The drawing under review shows one solid part. Ordinate dimensions are in mm from its lowest x, y, z. A direction names the side the tool comes from. Coordinates: 2 decimals unless noted, no trailing zeros. Order: outer loops, then holes, each group sorted by start corner. A loop starts at its lowest first (then second) coordinate and runs counter-clockwise, first axis right, second up.
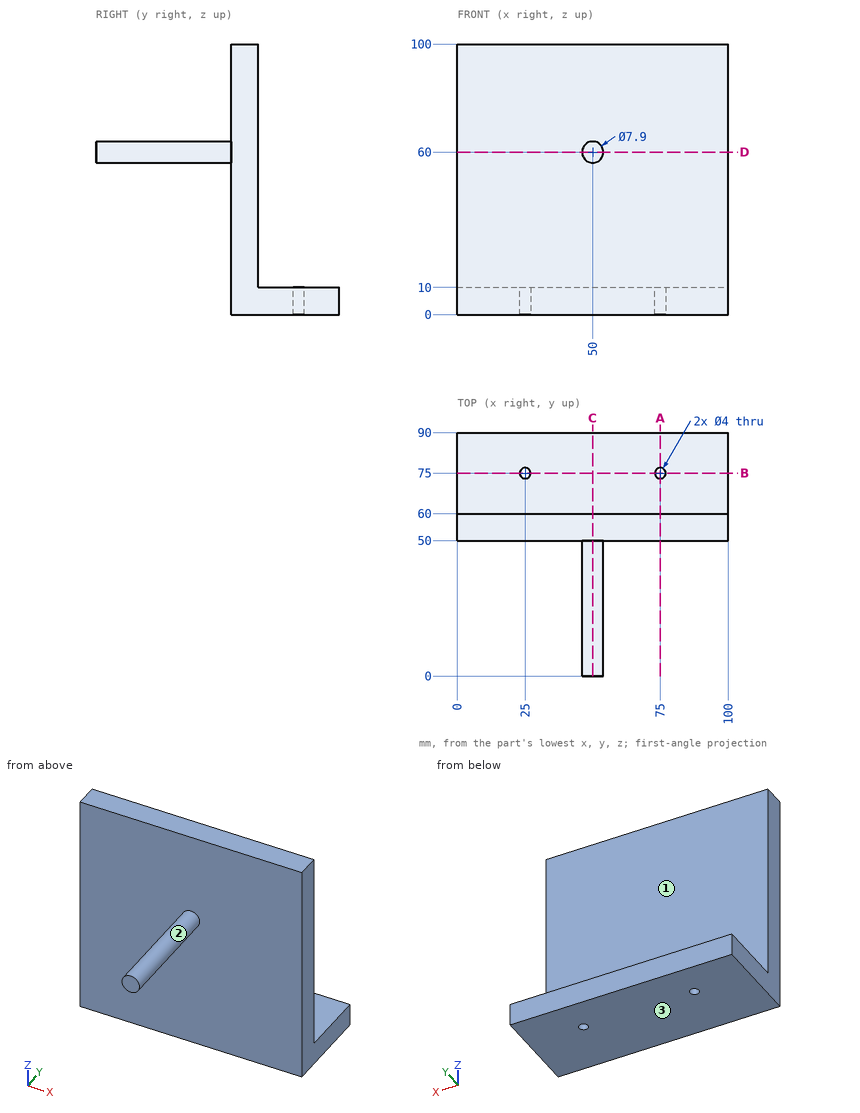
(1) Machinability: for the marked faces 1, 2 and 3, which of the approach directions +Z, -Z, +X, -X, +Y, -Y give a long, thin tool a straight path to every point of the face, cutting with its end or side? Answer none if there is none.
A:
face 1: +Z, +X, -X, +Y
face 2: -Y
face 3: -Z, +X, -X, +Y, -Y
(2) We need section B-B, the plane y = 75. Write out the cut boundary in (x, z).
A:
outline: (0, 0) - (23, 0) - (23, 10) - (0, 10) - close; (27, 0) - (73, 0) - (73, 10) - (27, 10) - close; (77, 0) - (100, 0) - (100, 10) - (77, 10) - close
(3) Wall thickness on probe 1 along Y at (x, z) = (75, 6); probe 2 along Z at (x, y) = (52, 82); probe 3 along Y at (x, z) = (48.5, 94): over which ranges is each line inside the solid? List them lowest first.
A:
probe 1: y = 50 to 73, 77 to 90
probe 2: z = 0 to 10
probe 3: y = 50 to 60
(4) We need section C-C, the plane x = 50. Write out the cut boundary in (y, z).
A:
outline: (0, 56.05) - (50, 56.05) - (50, 0) - (90, 0) - (90, 10) - (60, 10) - (60, 100) - (50, 100) - (50, 63.95) - (0, 63.95) - close
(5) For pin 1 Ø1 at (x, z) = (18.5, 77) entering from +Y, flat-tipped, find the tip position at first contact; note if it passes through.
A:
pin 1: stops at y = 60
(6) We need section A-A, the plane x = 75. Write out the cut boundary in (y, z), and give its area (3 significant figures).
A:
outline: (50, 0) - (73, 0) - (73, 10) - (60, 10) - (60, 100) - (50, 100) - close; (77, 0) - (90, 0) - (90, 10) - (77, 10) - close
area: 1,260 mm2
(7) We need section D-D, the plane z = 60. Write out the cut boundary in (x, y).
A:
outline: (0, 50) - (46.05, 50) - (46.05, 0) - (53.95, 0) - (53.95, 50) - (100, 50) - (100, 60) - (0, 60) - close
